Source: three-view drawing plus pictorial views. Frame: mm from the lowest corner of the part. A direction names the side the tool comes from. Coordinates: 2 decimals unless noted, no trailing zeros. Order: outer loops, then holes, each group sorted by start corner. A loop starts at its lowest first (then second) coordinate and runs counter-clockwise, first axis right, second up. Notation, with made-up numbers: M 88,58 L 96,58 A18 cw 96,86 Z; hole C -33.5,23 d5. An arc over 180 degrees is marked long. One line per question, with ' | ' between items.
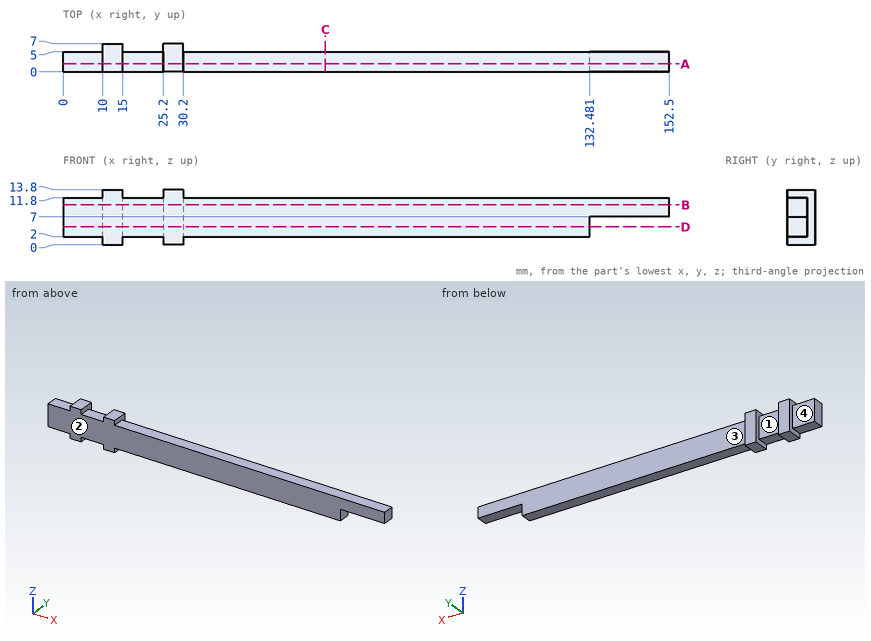
1. Pin query (flat end, axial travel): P1, Ø1, axis at y = 4, z = 2.5, coming from the -X side; P2, Ø4, axis at x = 57, y = 1.5, coming from the -Z side; P3, Ø1.5, axis at y = 3, z = 4.5, coming from the +X side; P4, Ø5, axis at x = 5.5, z = 5.5, coming from the +Y side. Return the tip coordinate at first contact, or that it passes through.
Response values:
P1: stops at x = 0 | P2: stops at z = 2 | P3: stops at x = 132.48 | P4: stops at y = 5
2. Section D-D, the plane z = 4.5. Output: boundary loops of the cut face in (x, y).
Response values:
outline: M 0,0 L 132.48,0 L 132.48,5 L 30.2,5 L 30.2,7 L 25.2,7 L 25.2,5 L 15,5 L 15,7 L 10,7 L 10,5 L 0,5 Z
3. Section A-A, the plane y = 2. Output: boundary loops of the cut face in (x, z), and give its area (3 significant figures).
Response values:
outline: M 0,2 L 10,2 L 10,0 L 15,0 L 15,2 L 25.2,2 L 25.2,0 L 30.2,0 L 30.2,2 L 132.48,2 L 132.48,7 L 152.5,7 L 152.5,11.8 L 30.2,11.8 L 30.2,13.8 L 25.2,13.8 L 25.2,11.8 L 15,11.8 L 15,13.8 L 10,13.8 L 10,11.8 L 0,11.8 Z | area: 1,430 mm^2
4. Access query for the marked faces 3 and 4. Directions: +Z, -Z, +X, -X, +Y, -Y. A direction counts if a zero-diameter tool reaches every point of the face in a straight line with its end or side. Return the directions, or none.
Response values:
face 3: +Z, -Z, +X, +Y | face 4: +Z, -Z, -X, +Y
5. Material intervals for line 1 (X direction, y = 2, z = 1); line 2 (Y direction, x = 122, z = 10.75); line 3 (X direction, y = 4.75, z = 6.75), sorted ascending. Write a range as [from, to].
Response values:
line 1: x = [10, 15], [25.2, 30.2] | line 2: y = [0, 5] | line 3: x = [0, 132.48]
6. Section C-C, the plane x = 66. Output: boundary loops of the cut face in (y, z).
Response values:
outline: M 0,2 L 5,2 L 5,11.8 L 0,11.8 Z
7. Section B-B, the plane z = 10. Output: boundary loops of the cut face in (x, y).
Response values:
outline: M 0,0 L 152.5,0 L 152.5,5 L 30.2,5 L 30.2,7 L 25.2,7 L 25.2,5 L 15,5 L 15,7 L 10,7 L 10,5 L 0,5 Z
8. Draft query along X for the marked faces 1 and 2. Return one class per face: pulls with the +X half, pulls with the -X half, needs draft (parallel to the pull), parting line crosses it, or undercut.
Response values:
face 1: undercut | face 2: needs draft
